Source: CAD feature listing. Evaluate the final solid. Frame: model axes, mm. A direction names the side the tool comes from. Give positions to 0.01 mm unless a question says otherwise; leave off trailing zeros. Order: outer loops, then holes, each group sorted by start corner. A loop starts at its lowest first (then second) coordinate and runs counter-clockwise, first axis right, second up.
1) Section B-B, the plane x = -20. Return loops of the section in (y, z), plus the area to 3 significant figures.
2) Access query for faces 1 (the face through (-18.55, 3.5, 2.1)), 2 (the face through (-21.45, 3.5, 9.9)), 3 (the face through (1.45, 3.5, 17.8)). Directions: +Z, -Z, +X, -X, +Y, -Y. A direction counts if a zero-diameter tool reaches every point of the face in a straight line with its end or side. Return the directions, or none.
3) Section D-D, the plane z = 11.75. Return loops of the section in (x, y).
4) Section C-C, the plane y = 1.45. Return loops of the section in (x, z).
5) First-contact query: P1, Ø4, axis at x = -11.5, z = 6.5, coming from the -Y side; P2, Ø0.8, axis at y = 3.5, z = 18.5, coming from the +X side; P3, Ø0.5, axis at y = 3.5, z = 2.5, coming from the -X side; P4, Ø3.5, axis at x = -15.5, z = 13.5, coming from the +Y side. Flat tips, straight axial feed; report the tip coordinate or a pass-through.
6) Material intervals for line 1 (X direction, y = 1.5, z = 15); line 2 (Z direction, x = -10, y = 3.1); line 3 (Z direction, x = -8.75, y = 1.6), sorted ascending.
7) Section A-A, the plane z = 5. Return loops of the section in (x, y), plus the area to 3 significant figures.
8) Draft query along Z for faces 4 (the face through (-21.6, 2.03, 4.93)), 5 (the face through (3, 3, 10)). Return one class per face: released by +Z, released by -Z, zero draft, split by the parting line, or undercut.
```python
from build123d import *

# Parameters (mm, degrees)
MAIN_DEPTH                 = 20
ESQUISSE2_R                = 1.6
TOPHOLE_DEPTH              = 5
R_P_TITION_LIN_AIRE1_COUNT = 3
R_P_TITION_LIN_AIRE1_PITCH = 10


with BuildPart() as part:
    # Esquisse1 → Main (new body)
    with BuildSketch(Plane.XY):
        Polygon((-5, 0), (-5, 3), (-1.45, 3), (-1.45, 4), (1.45, 4), (1.45, 3), (5, 3), (5, 0), align=None)
    main = extrude(amount=MAIN_DEPTH)

    # Esquisse2 → TopHole (cut, through all)
    with BuildSketch(Plane(origin=(0, 4, 0), x_dir=(1, 0, 0), z_dir=(0, 1, 0))):
        with Locations((0, -5)):
            Circle(ESQUISSE2_R)
        with Locations((0, -15)):
            Circle(ESQUISSE2_R)
    tophole = extrude(amount=-TOPHOLE_DEPTH, mode=Mode.SUBTRACT)

    # Répétition linéaire1: Main, TopHole ×3
    with Locations(*[(-i * R_P_TITION_LIN_AIRE1_PITCH, 0, 0) for i in range(1, R_P_TITION_LIN_AIRE1_COUNT)]):
        add(main)
        add(tophole, mode=Mode.SUBTRACT)


solid = part.part
```
From the geometry:
1. outline: (0, 0) - (4, 0) - (4, 3.4) - (0, 3.4) - close; (0, 6.6) - (4, 6.6) - (4, 13.4) - (0, 13.4) - close; (0, 16.6) - (4, 16.6) - (4, 20) - (0, 20) - close
1. area: 54.4 mm2
2. face 1: +Z, -Z, +Y
2. face 2: +Z, -Z, -X, +Y
2. face 3: +Z, -Z, +X, +Y
3. outline: (-25, 0) - (5, 0) - (5, 3) - (1.45, 3) - (1.45, 4) - (-1.45, 4) - (-1.45, 3) - (-8.55, 3) - (-8.55, 4) - (-11.45, 4) - (-11.45, 3) - (-18.55, 3) - (-18.55, 4) - (-21.45, 4) - (-21.45, 3) - (-25, 3) - close
4. outline: (-25, 0) - (5, 0) - (5, 20) - (-25, 20) - close; hole circle Ø3.2 at (-20, 5); hole circle Ø3.2 at (-20, 15); hole circle Ø3.2 at (-10, 5); hole circle Ø3.2 at (-10, 15); hole circle Ø3.2 at (0, 5); hole circle Ø3.2 at (0, 15)
5. P1: stops at y = 0
5. P2: stops at x = 1.45
5. P3: stops at x = -21.45
5. P4: stops at y = 3
6. line 1: x = -25 to -21.6, -18.4 to -11.6, -8.4 to -1.6, 1.6 to 5
6. line 2: z = 0 to 3.4, 6.6 to 13.4, 16.6 to 20
6. line 3: z = 0 to 4, 6 to 14, 16 to 20
7. outline: (-25, 0) - (-21.6, 0) - (-21.6, 3) - (-25, 3) - close; (-18.4, 0) - (-11.6, 0) - (-11.6, 3) - (-18.4, 3) - close; (-8.4, 0) - (-1.6, 0) - (-1.6, 3) - (-8.4, 3) - close; (1.6, 0) - (5, 0) - (5, 3) - (1.6, 3) - close
7. area: 61.2 mm2
8. face 4: undercut
8. face 5: zero draft
